Build history of the part. All positions in model axes, mm. Give positions to 0.01 mm unless a question says otherwise; leave off trailing zeros. Write each loop counter-clockwise with the first axis right and the second up, starting at its lowest first coordinate (ties: lowest second). Pieces come first, ordered by that corner, then holes. Notation, with made-up numbers: (-12.5, 47.25) - (19.5, 47.25) arc R28 ccw to (19.5, 71.25) - close; hole circle Ø8 at (52.5, 0). An arc over 180 degrees is marked (long way). Use one line per item in the form item = value. Start each with the question number.
from build123d import *

# Parameters (mm, degrees)
F0_W     = 82.55
F0_H     = 31.75
F0_R     = 3.429
F0_R_2   = 5.715
F1_DEPTH = 6.35
F2_R     = 6.35
F3_R     = 1.27


with BuildPart() as f1:
    # F0 (on Top) → F1 (new body)
    with BuildSketch(Plane.XY):
        Rectangle(F0_W, F0_H)
        with Locations((-25.4, 0)):
            Circle(F0_R, mode=Mode.SUBTRACT)
        Circle(F0_R_2, mode=Mode.SUBTRACT)
        with Locations((25.4, 0)):
            Circle(F0_R, mode=Mode.SUBTRACT)
    extrude(amount=F1_DEPTH)

    # F2
    f2_edges = [f1.edges().sort_by_distance(p)[0] for p in [
        (-41.275, -15.875, 3.175),
        (41.275, -15.875, 3.175),
        (41.275, 15.875, 3.175),
        (-41.275, 15.875, 3.175),
    ]]
    fillet(f2_edges, radius=F2_R)

    # F3
    f3_edges = [f1.edges().sort_by_distance(p)[0] for p in [
        (0, -15.875, 6.35),
        (0, -15.875, 0),
    ]]
    fillet(f3_edges, radius=F3_R)


solid = f1.part
(1) Two-plate mould, pull along Y, no slides. Class faces 1 (the flat face through (0, 15.875, 3)), 2 (the flat face through (0, -15.875, 3)), 3 (the cylindrical face through (21.974, 0.151, 3.131)): +Y half, -Y half, draft (parallel to the pull), parting line (faces both ways), or undercut.
(2) Pin check, flat tip, straight feed: pin 1 Ø4 at (x, y) = (-25.4, 0) entering from +Z. Stop position of the tip, or through.
(3) Cut at A-A, the plane x = 25.4. Give the cut face in (y, z) (3 decimals), then the cut area to 3 significant figures.
(4) Cut at B-B, the plane z = 2. Give the cut face in (x, y) (3 decimals).
(5) Cut at C-C, the plane y = 0. Give the cut face in (x, z) (3 decimals).
(6) Wall check: line 1 (Y direction, x = 0, z = 2) (3 decimals); line 2 (X direction, y = -0.5, z = 3.5) (3 decimals); line 3 (Y direction, x = -3, z = 1.75) (3 decimals). Give the ranges that are in metal, low to high. Write a range as from..to.
(7) Cut at D-D, the plane x = 0. Give the cut face in (y, z) (3 decimals), then the cut area to 3 significant figures.
Solution:
q1.face_1 = +Y half
q1.face_2 = -Y half
q1.face_3 = undercut
q2.pin_1 = through
q3.outline = (-15.875, 1.27) arc R1.27 ccw to (-14.605, 0) - (-3.429, 0) - (-3.429, 6.35) - (-14.605, 6.35) arc R1.27 ccw to (-15.875, 5.08) - close; (3.429, 0) - (14.605, 0) arc R1.27 ccw to (15.875, 1.27) - (15.875, 5.08) arc R1.27 ccw to (14.605, 6.35) - (3.429, 6.35) - close
q3.area = 157 mm2
q4.outline = (-41.275, -9.525) arc R6.35 ccw to (-34.925, -15.875) - (34.925, -15.875) arc R6.35 ccw to (41.275, -9.525) - (41.275, 9.525) arc R6.35 ccw to (34.925, 15.875) - (-34.925, 15.875) arc R6.35 ccw to (-41.275, 9.525) - close; hole circle Ø6.858 at (-25.4, 0); hole circle Ø11.43 at (0, 0); hole circle Ø6.858 at (25.4, 0)
q5.outline = (-41.275, 1.27) arc R1.27 ccw to (-40.005, 0) - (-28.829, 0) - (-28.829, 6.35) - (-40.005, 6.35) arc R1.27 ccw to (-41.275, 5.08) - close; (-21.971, 0) - (-5.715, 0) - (-5.715, 6.35) - (-21.971, 6.35) - close; (5.715, 0) - (21.971, 0) - (21.971, 6.35) - (5.715, 6.35) - close; (28.829, 0) - (40.005, 0) arc R1.27 ccw to (41.275, 1.27) - (41.275, 5.08) arc R1.27 ccw to (40.005, 6.35) - (28.829, 6.35) - close
q6.line_1 = -15.875..-5.715, 5.715..15.875
q6.line_2 = -41.275..-28.792, -22.008..-5.693, 5.693..22.008, 28.792..41.275
q6.line_3 = -15.875..-4.864, 4.864..15.875
q7.outline = (-15.875, 1.27) arc R1.27 ccw to (-14.605, 0) - (-5.715, 0) - (-5.715, 6.35) - (-14.605, 6.35) arc R1.27 ccw to (-15.875, 5.08) - close; (5.715, 0) - (14.605, 0) arc R1.27 ccw to (15.875, 1.27) - (15.875, 5.08) arc R1.27 ccw to (14.605, 6.35) - (5.715, 6.35) - close
q7.area = 128 mm2
